Geometry check sheet. Reference: the model listing, model coordinates, mm. A direction names the side the tool comes from. Round coordinates to 2 decimals unless told otherwise and drop trailing zeros. Write each loop counter-clockwise with the first axis right and the second up, starting at its lowest first coordinate (ties: lowest second). Pieces come first, ordered by that corner, then holes. Notation, with made-up numbers: M 76.5,69.25 L 124.5,69.25 A26 ccw 124.5,89.25 Z; hole C 86.25,-26 d8. An arc over 180 degrees is marked long. Put each result on its own line as item: value. Start each with the question number.
(1) Section check C-C on x = -309. Record the cut outline in (y, z).
(2) Section check B-B on z = 195. Record the cut outline in (x, y).
(3) Section check A-A on x = -521.5. Record the cut outline in (y, z).
(4) Tool access check on faces 4 (the flat face through (-4, 14851, 0)), 5 (the flat face through (-151, 14800, 123)), 6 (the cylindrical face through (-355.89, 14970.77, 123.25)), 7 (the flat face through (-11, 14750, -67)). Record the directions out of +Z, -Z, +X, -X, +Y, -Y that give a thin tool (end or side, any length) a straight path to the whole face; none if there is none.
(5) Mould release check, pull along Y, two halves, no side actions. Record for faces 1 (the flat face through (-11, 14675, 131)), 2 (the flat face through (-250, 14775, 123)), 3 (the flat face through (-4, 14851, 250)): pulls with the +Y half, pulls with the -Y half, needs draft (parallel to the pull), parting line crosses it, or undercut.
(6) Gauge pin test, flat ends, axial feed: pin 1 (3 mm diameter, centred on y = 14919.5, z = 66.5, fed in from +X); pin 2 (1.5 mm diameter, centred on x = 444.5, z = -122, fed in from -Y); pin 3 (8 mm diameter, centred on x = -338, z = 271, fed in from +Y). Record the tip position at first contact, or that the pin passes through.
(7) Material ranges on probe 1 along Y at (x, z) = (-8, -37); probe 2 along Z at (x, y) = (-142.5, 14769.5); probe 3 along Y at (x, z) = (-426.5, 79.5), recorded low to high.
(8) Section check D-D on z = 325.5. Record the cut outline in (x, y), then the cut area to 3 significant figures.
from build123d import *

# Parameters (mm, degrees)
F0_W     = 200
F0_H     = 50
F0_W_2   = 50
F1_DEPTH = 250
F2_W     = 1536.897368713
F2_H     = 893.9969116518
F3_DEPTH = 80
F4_W     = 1506.897368713
F4_H     = 863.9969116518
F5_DEPTH = 5


with BuildPart() as f1:
    # F0 (on Top) → F1 (new body)
    with BuildSketch(Plane.XY):
        with BuildLine():
            ThreePointArc((652.5786238231, 14970.7837516855), (-0.5294510276, 14984.9999906467), (-653.6365196693, 14970.7376004041))
            Line((-653.6365196696, 14970.7376004041), (-653.2003257959, 14960.7471181883))
            ThreePointArc((-653.200325796, 14960.7471181883), (-351.6715336626, 14970.8701194156), (-50, 14974.9165273133))
            ThreePointArc((-50, 14974.9165273133), (-25.0000348384, 14974.9791318138), (0, 14975))
            ThreePointArc((0, 14975), (25.0000348384, 14974.9791318138), (50, 14974.9165273133))
            ThreePointArc((50, 14974.9165273133), (351.1425816533, 14970.8825353534), (652.1431359193, 14960.7932386713))
            Line((652.1431359193, 14960.7932386713), (652.5786238231, 14970.7837516855))
        make_face()
        with BuildLine():
            ThreePointArc((0, 14975), (-25.0000348384, 14974.9791318138), (-50, 14974.9165273133))
            Line((-50, 14974.9165273133), (-50, 14800))
            Line((-50, 14800), (0, 14800))
            Line((0, 14800), (0, 14975))
        make_face()
        with BuildLine():
            Line((50, 14800), (50, 14974.9165273133))
            ThreePointArc((50, 14974.9165273133), (25.0000348384, 14974.9791318138), (0, 14975))
            Line((0, 14975), (0, 14800))
            Line((0, 14800), (50, 14800))
        make_face()
        with Locations((-150, 14775)):
            Rectangle(F0_W, F0_H)
        with Locations((-25, 14775)):
            Rectangle(F0_W_2, F0_H)
        with Locations((25, 14775)):
            Rectangle(F0_W_2, F0_H)
        with Locations((150, 14775)):
            Rectangle(F0_W, F0_H)
    extrude(amount=F1_DEPTH)

    # F2 (on face) → F3 (join)
    with BuildSketch(Plane.XZ.offset(-14750)):
        with Locations((0, 125)):
            Rectangle(F2_W, F2_H)
    extrude(amount=F3_DEPTH)

    # F4 (on face) → F5 (cut)
    with BuildSketch(Plane.XZ.offset(-14670)):
        with Locations((0, 125)):
            Rectangle(F4_W, F4_H)
    extrude(amount=-F5_DEPTH, mode=Mode.SUBTRACT)


solid = f1.part
Answers follow:
1. outline: M 14670,-322 L 14750,-322 L 14750,572 L 14670,572 L 14670,557 L 14675,557 L 14675,-307 L 14670,-307 Z; M 14971.81,0 L 14981.81,0 L 14981.81,250 L 14971.81,250 Z
2. outline: M -768.45,14670 L -753.45,14670 L -753.45,14675 L 753.45,14675 L 753.45,14670 L 768.45,14670 L 768.45,14750 L 250,14750 L 250,14800 L 50,14800 L 50,14974.92 A14975 cw 652.14,14960.79 L 652.58,14970.78 A14985 ccw -653.64,14970.74 L -653.2,14960.75 A14975 cw -50,14974.92 L -50,14800 L -250,14800 L -250,14750 L -768.45,14750 Z
3. outline: M 14670,-322 L 14750,-322 L 14750,572 L 14670,572 L 14670,557 L 14675,557 L 14675,-307 L 14670,-307 Z; M 14965.92,0 L 14975.92,0 L 14975.92,250 L 14965.92,250 Z
4. face 4: -Z, +X, -X, +Y
4. face 5: +Z, -Z, -X
4. face 6: +Z, -Z
4. face 7: none
5. face 1: pulls with the -Y half
5. face 2: undercut
5. face 3: needs draft
6. pin 1: stops at x = 50
6. pin 2: stops at y = 14675
6. pin 3: stops at y = 14750
7. probe 1: y = 14675 to 14750
7. probe 2: z = 0 to 250
7. probe 3: y = 14675 to 14750, 14968.93 to 14978.93
8. outline: M -768.45,14670 L -753.45,14670 L -753.45,14675 L 753.45,14675 L 753.45,14670 L 768.45,14670 L 768.45,14750 L -768.45,14750 Z
8. area: 115,000 mm^2
